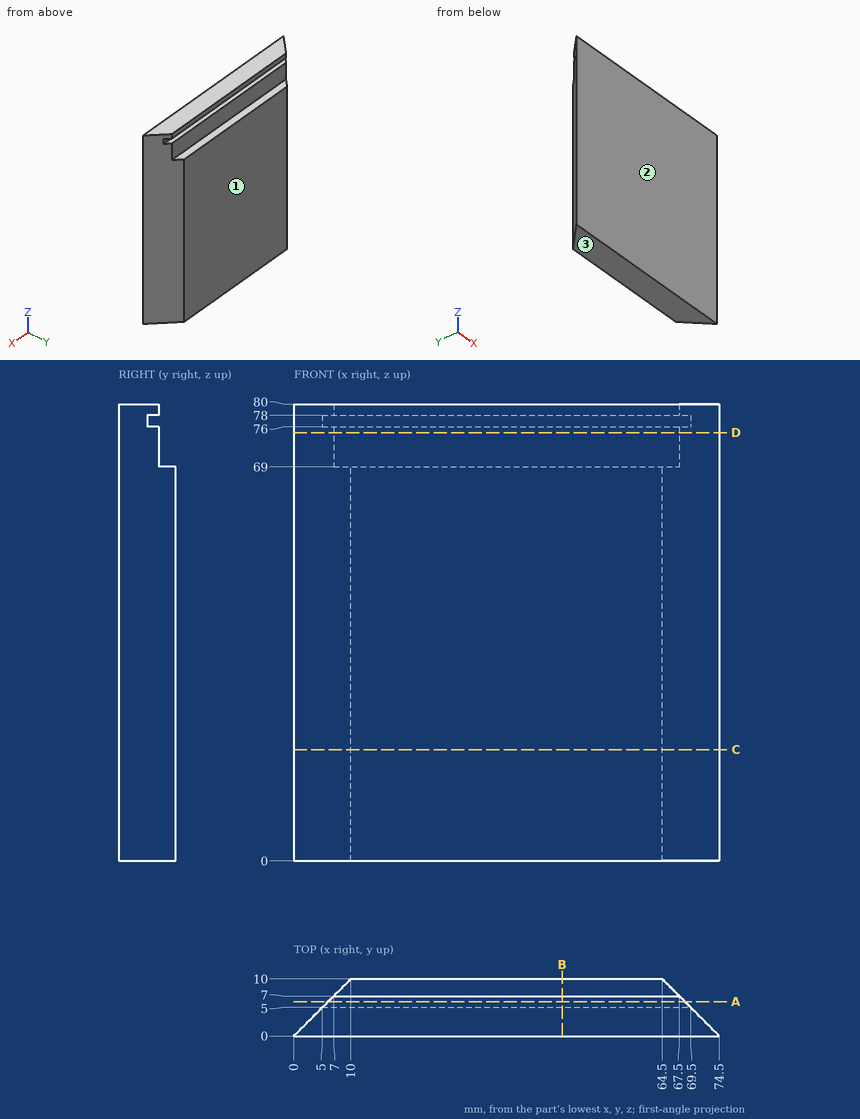
For this review, use the dimensioned drawing (mm, ordinates from the lowest corner) and the shaded views. Round coordinates to 2 decimals unless told otherwise and drop trailing zeros. Write each loop counter-clockwise with the first axis right and the second up, starting at its lowest first coordinate (ties: lowest second). Pieces come first, ordered by that corner, then holes. Notation, with made-up numbers: (68, 72.5) -> (110, 72.5) arc R23 ccw to (110, 111.5) -> close; hole circle Ø1 at (48, -32). An arc over 180 degrees is marked (long way). One line per item, written item: value. Start each with the question number.
Q1. Add section C-C (z = 19.5). Give the boundary of the cut face in (x, y), then the cut area to 3 significant figures.
Q2. Add section D-D (z = 75). Give the boundary of the cut face in (x, y).
Q3. Add section A-A (y = 6). Give the boundary of the cut face in (x, z), then the cut area to 4 significant figures.
Q4. Add section B-B (x = 47). Give the boundary of the cut face in (y, z).
Q5. The part is to be moulded in two halves that separate along Y. For the marked faces 1, 2 and 3, say which applies: pulls with the +Y half, pulls with the -Y half, needs draft (parallel to the pull), parting line crosses it, or undercut.
Q6. To check wall thickness, follow probe 1 along Z at (x, y) = (53, 6.5); probe 2 along Y at (x, z) = (33.5, 74); probe 3 along X at (y, z) = (1.25, 72). State the ranges of each line that lie inside material, in increasing order.
Q7. Insertion check: P1, Ø2, axis at y = 4.5, z = 11, coming from the -X side; P2, Ø1.6, axis at x = 31.5, z = 77.5, coming from the +Y side; P3, Ø6, axis at y = 4.5, z = 69.5, coming from the -X side. Each pin has a flat end and moves straight along its axis. Give the tip position at first contact, or say it passes through.
Response:
1. outline: (0, 0) -> (74.5, 0) -> (64.5, 10) -> (10, 10) -> close
1. area: 645 mm^2
2. outline: (0, 0) -> (74.5, 0) -> (67.5, 7) -> (7, 7) -> close
3. outline: (6, 0) -> (68.5, 0) -> (68.5, 76) -> (6, 76) -> close; (6, 78) -> (68.5, 78) -> (68.5, 80) -> (6, 80) -> close
3. area: 4,875 mm^2
4. outline: (0, 0) -> (10, 0) -> (10, 69) -> (7, 69) -> (7, 76) -> (5, 76) -> (5, 78) -> (7, 78) -> (7, 80) -> (0, 80) -> close
5. face 1: pulls with the +Y half
5. face 2: pulls with the -Y half
5. face 3: needs draft
6. probe 1: z = 0 to 76, 78 to 80
6. probe 2: y = 0 to 7
6. probe 3: x = 1.25 to 73.25
7. P1: stops at x = 3.5
7. P2: stops at y = 7
7. P3: stops at x = 1.5
